For this review, take the finished solid that the model builds, in its own axes (mm). A direction names the side the tool comes from. Give positions to 0.01 mm unless a question says otherwise; leave off trailing zeros. Loops run counter-clockwise (first coordinate to the right, second up) from the corner with the lowest first, then second, coordinate; pieces in that order, holes last. Notation, with made-up numbers: (15, 80.25) -> (59, 80.25) arc R19 ccw to (59, 104.25) -> close; hole circle Ø5 at (32, 40). An arc over 180 degrees is marked (long way). Write each question's results on one line, items separated by ' | '. Start each with the question number.
```python
from build123d import *

# Parameters (mm, degrees)
SKETCH1_R           = 22.5
BOSS_EXTRUDE1_DEPTH = 55
SKETCH2_R           = 5
CUT_EXTRUDE1_DEPTH  = 10
SKETCH3_R           = 5
CUT_EXTRUDE2_DEPTH  = 10


with BuildPart() as part:
    # Sketch1 → Boss-Extrude1 (new body)
    with BuildSketch(Plane(origin=(0, 0, 0), x_dir=(1, 0, 0), z_dir=(0, 1, 0))):
        Circle(SKETCH1_R)
    extrude(amount=BOSS_EXTRUDE1_DEPTH)

    # Sketch2 → Cut-Extrude1 (cut)
    with BuildSketch(Plane(origin=(0, 55, 0), x_dir=(1, 0, 0), z_dir=(0, 1, 0))):
        Circle(SKETCH2_R)
    extrude(amount=-CUT_EXTRUDE1_DEPTH, mode=Mode.SUBTRACT)

    # Sketch3 → Cut-Extrude2 (cut)
    with BuildSketch(Plane.XZ):
        Circle(SKETCH3_R)
    extrude(amount=-CUT_EXTRUDE2_DEPTH, mode=Mode.SUBTRACT)


solid = part.part
```
1. We need section A-A (x = 0). Write out the cut boundary in (y, z).
2. Wall thickness on L1, parallel to Z at x = 0, y = 7.5; L2, parallel to Z at x = -3, y = 52; L3, parallel to X at y = 34.5, z = 1.5: over which ranges is each line inside the solid? List them lowest first.
3. We need section C-C (y = 12). Write out the cut boundary in (x, z).
4. Draft analysis for pull direction X (two halves, no side actions). For faces 4 (the cylindrical face through (10.382, 27.115, 19.961)), 5 (the flat face through (0, 45, 0)), 6 (the flat face through (-0.3, 0, -5.3)), state which applies: released by +X, released by -X, zero draft, split by the parting line, or undercut.
5. We need section B-B (z = 0). Write out the cut boundary in (x, y), plus the area to 4 significant figures.
6. Machinability: for faces 1 (the flat face through (-0.3, 55, -5.3)), 2 (the cylindrical face through (-1.08, 50.07, 4.88)), 3 (the cylindrical face through (-1.08, 4.93, -4.88)), which of the approach directions +Z, -Z, +X, -X, +Y, -Y give a long, thin tool a straight path to every point of the face, cutting with its end or side? Answer none if there is none.
7. For pin 1 Ø6 at (x, z) = (0, 0) entering from -Y; pin 2 Ø2 at (y, z) = (22.5, 14.5) entering from +X; pin 3 Ø1 at (x, z) = (11, -2) entering from -Y; pin 4 Ø3 at (y, z) = (7, 5) entering from +X, all flat-tipped, find the tip position at first contact; note any pin that passes through.
8. We need section D-D (x = 18). Write out the cut boundary in (y, z).
Response:
1) outline: (0, -22.5) -> (55, -22.5) -> (55, -5) -> (45, -5) -> (45, 5) -> (55, 5) -> (55, 22.5) -> (0, 22.5) -> (0, 5) -> (10, 5) -> (10, -5) -> (0, -5) -> close
2) L1: z = -22.5 to -5, 5 to 22.5 | L2: z = -22.3 to -4, 4 to 22.3 | L3: x = -22.45 to 22.45
3) outline: circle Ø45 at (0, 0)
4) face 4: split by the parting line | face 5: undercut | face 6: zero draft
5) outline: (-22.5, 0) -> (-5, 0) -> (-5, 10) -> (5, 10) -> (5, 0) -> (22.5, 0) -> (22.5, 55) -> (5, 55) -> (5, 45) -> (-5, 45) -> (-5, 55) -> (-22.5, 55) -> close | area: 2,275 mm2
6) face 1: +Z, -Z, +X, -X, +Y | face 2: +Y | face 3: -Y
7) pin 1: stops at y = 10 | pin 2: stops at x = 18 | pin 3: stops at y = 0 | pin 4: stops at x = 22.23
8) outline: (0, -13.5) -> (55, -13.5) -> (55, 13.5) -> (0, 13.5) -> close
